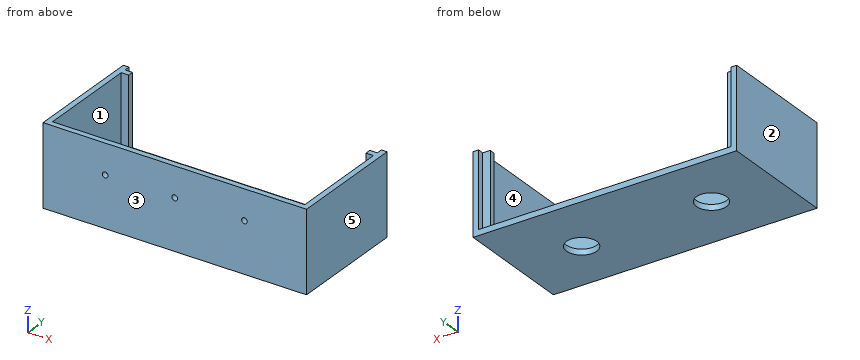
from build123d import *

# Parameters (mm, degrees)
F0_R     = 8
F1_DEPTH = 3
F2_W     = 3
F2_H     = 3
F2_W_2   = 134
F3_DEPTH = 40
F4_W     = 3
F4_H     = 40
F5_DEPTH = 134
F6_W     = 126
F6_H     = 3
F7_DEPTH = 40
F8_R     = 1.5
F9_DEPTH = 3


with BuildPart() as f1:
    # F0 (on Top) → F1 (new body)
    with BuildSketch(Plane.XY):
        Polygon((-60, 33.034884), (-80, 33.034884), (-80, 18.034884), (-80, 0.034884), (-80, -2.965116), (-80, -17.965116), (-80, -29.965116), (60, -29.965116), (60, -24.965116), (60, -14.965116), (60, -9.965116), (60, -4.965116), (60, 0.034884), (60, 18.034884), (60, 33.034884), (40, 33.034884), (20, 33.034884), (0, 33.034884), (-20, 33.034884), (-40, 33.034884), align=None)
        with Locations((25, -0.468963)):
            Circle(F0_R, mode=Mode.SUBTRACT)
        with Locations((-45, 1.034884)):
            Circle(F0_R, mode=Mode.SUBTRACT)
    extrude(amount=F1_DEPTH)

    # F2 (on face) → F3 (join)
    with BuildSketch(Plane.XY.offset(3)):
        with Locations((-78.5, -28.465116)):
            Rectangle(F2_W, F2_H)
        with Locations((-10, -28.465116)):
            Rectangle(F2_W_2, F2_H)
        Polygon((-80, 30.034884), (-80, -26.965116), (-77, -26.965116), (-77, 33.034884), (-80, 33.034884), align=None)
        with Locations((58.5, -28.465116)):
            Rectangle(F2_W, F2_H)
        Polygon((57, 33.034884), (57, -26.965116), (60, -26.965116), (60, 30.034884), (60, 33.034884), align=None)
    extrude(amount=F3_DEPTH)

    # F4 (on face) → F5 (join)
    with BuildSketch(Plane.YZ.offset(-77)):
        with Locations((28.334884, 23)):
            Rectangle(F4_W, F4_H)
    extrude(amount=F5_DEPTH)

    # F6 (on face) → F7 (cut)
    with BuildSketch(Plane.XY.offset(43)):
        with Locations((-10, 28.334884)):
            Rectangle(F6_W, F6_H)
    extrude(amount=-F7_DEPTH, mode=Mode.SUBTRACT)

    # F8 (on face) → F9 (cut)
    with BuildSketch(Plane(origin=(0, -26.965116, 0), x_dir=(-1, 0, 0), z_dir=(0, 1, 0))):
        with Locations((47, 26.988985)):
            Circle(F8_R)
        with Locations((-27, 26.988985)):
            Circle(F8_R)
        with Locations((10, 26.988985)):
            Circle(F8_R)
    extrude(amount=-F9_DEPTH, mode=Mode.SUBTRACT)


solid = f1.part
For this review, take the finished solid that the model builds, in its own axes (mm). Face numbers are marked on the shaded views. A direction names the side the tool comes from. Give positions to 0.01 mm unless a question says otherwise; leave off trailing zeros. Write each loop counter-clockwise with the first axis right and the second up, starting at its lowest first coordinate (ties: lowest second). Pieces come first, ordered by that corner, then holes. Notation, with made-up numbers: (-39.75, 13.25) -> (-27.75, 13.25) arc R19 ccw to (-27.75, 28.25) -> close; hole circle Ø10 at (-37.5, 16.5). An arc over 180 degrees is marked (long way). Use CSV: the item, a comma, the result in double quotes.
Q1. Mouldability with a two-part tool opening along Y and no side actions: class the marked faces 3, 4 and 5 as pulls with the +Y half, pulls with the -Y half, needs draft (parallel to the pull), parting line crosses it, or undercut.
Conclusion:
face 3,"pulls with the -Y half"
face 4,"undercut"
face 5,"needs draft"
Q2. Take a section at D-D, the plane x = -7. Write out the cut boundary in (y, z), then the cut area to 3 significant figures.
Conclusion:
outline,"(-29.97, 0) -> (33.03, 0) -> (33.03, 3) -> (-26.97, 3) -> (-26.97, 43) -> (-29.97, 43) -> close"
area,"309 mm2"
Q3. Tool access review of the marked faces 1 and 2: name each direction out of +Z, -Z, +X, -X, +Y, -Y from which nothing blocks a thin tool from reaching the whole face with its end or side.
Conclusion:
face 1,"+Z"
face 2,"+Z, -Z, -X, +Y, -Y"
Q4. Take a section at C-C, the plane z = 16. Write out the cut boundary in (x, y).
Conclusion:
outline,"(-80, -29.97) -> (60, -29.97) -> (60, 33.03) -> (57, 33.03) -> (57, 29.83) -> (53, 29.83) -> (53, 26.83) -> (57, 26.83) -> (57, -26.97) -> (-77, -26.97) -> (-77, 26.83) -> (-73, 26.83) -> (-73, 29.83) -> (-77, 29.83) -> (-77, 33.03) -> (-80, 33.03) -> close"
Q5. Take a section at B-B, the plane y = 17. Write out the cut boundary in (x, z), then the cut area to 3 significant figures.
Conclusion:
outline,"(-80, 0) -> (60, 0) -> (60, 43) -> (57, 43) -> (57, 3) -> (-77, 3) -> (-77, 43) -> (-80, 43) -> close"
area,"660 mm2"
Q6. Take a section at A-A, the plane x = 27. Write out the cut boundary in (y, z), then the cut area to 3 significant figures.
Conclusion:
outline,"(-29.97, 0) -> (-8.21, 0) -> (-8.21, 3) -> (-26.97, 3) -> (-26.97, 25.49) -> (-29.97, 25.49) -> close; (-29.97, 28.49) -> (-26.97, 28.49) -> (-26.97, 43) -> (-29.97, 43) -> close; (7.28, 0) -> (33.03, 0) -> (33.03, 3) -> (7.28, 3) -> close"
area,"254 mm2"
Q7. For P1, Ø14.5, axis at x = -45, y = 1.03, coming from the -Z side; P2, Ø4, axis at x = 27, z = 26.99, coming from the +Y side; P3, Ø1, axis at x = 41, y = 24, coming from the +Z side; P4, Ø1.2, axis at x = 54.5, z = 28, coming from the +Y side, all flat-tipped, find the tip position at first contact; note any pin that passes through.
Conclusion:
P1,"through"
P2,"y = -26.97"
P3,"z = 3"
P4,"y = 29.83"
Q8. To check wall thickness, follow probe 1 along Y at (x, z) = (-45, 1.35); probe 2 along X at (y, z) = (2, 10); probe 3 along Y at (x, z) = (25, 1). State the ranges of each line that lie inside material, in increasing order. Write a range as [from, to].
Conclusion:
probe 1,"[-29.97, -6.97], [9.03, 33.03]"
probe 2,"[-80, -77], [57, 60]"
probe 3,"[-29.97, -8.47], [7.53, 33.03]"
